Part model, mm, in its own coordinate system. Face numbers are marked on the shaded views. A direction names the side the tool comes from. Give positions to 0.01 mm unless a question says otherwise; leave off trailing zeros. Write each loop counter-clockwise with the first axis right and the second up, starting at its lowest first coordinate (ties: lowest second). Pieces come first, ordered by that corner, then holes. Notation, with made-up numbers: (9, 78) - (26, 78) arc R20 cw to (26, 115) - close; hole circle Ø11 at (-25, 27). An arc over 180 degrees is marked (long way). Answer as a JSON object with one key per item and string values. Group by question number.
```python
from build123d import *

# Parameters (mm, degrees)
SKETCH1_W                     = 196.85
SKETCH1_H                     = 152.4
SKETCH1_W_2                   = 146.05
SKETCH1_H_2                   = 101.6
BOSS_EXTRUDE1_DEPTH           = 1.5875
EDGE_FLANGE1_STRIP_W          = 26.35
EDGE_FLANGE1_STRIP_H          = 1.5875
EDGE_FLANGE1_STRIP_CUT_DEPTH  = 152.4
EDGE_FLANGE1_DEPTH            = 152.4
EDGE_FLANGE2_STRIP_W          = 26.35
EDGE_FLANGE2_STRIP_H          = 1.5875
EDGE_FLANGE2_STRIP_CUT_DEPTH  = 152.4
EDGE_FLANGE2_DEPTH            = 152.4
SKETCH16_W                    = 146.05
SKETCH16_H                    = 101.6
CUT_EXTRUDE1_DEPTH            = 1.5875
SKETCH17_W                    = 31.75
SKETCH17_H                    = 114.3
CUT_EXTRUDE2_DEPTH            = 1.5875
SKETCH25_W                    = 1.5875
SKETCH25_H                    = 101.6
CUT_EXTRUDE3_DEPTH            = 0.0254
EDGE_FLANGE5_STRIP_W          = 26.35
EDGE_FLANGE5_STRIP_H          = 1.5875
EDGE_FLANGE5_STRIP_CUT_DEPTH  = 25.4
EDGE_FLANGE5_RELIEF_W         = 27.14375
EDGE_FLANGE5_RELIEF_H         = 0.79375
EDGE_FLANGE5_RELIEF_CUT_DEPTH = 1.5875
EDGE_FLANGE5_DEPTH            = 25.4
EDGE_FLANGE6_STRIP_W          = 26.35
EDGE_FLANGE6_STRIP_H          = 1.5875
EDGE_FLANGE6_STRIP_CUT_DEPTH  = 25.4
EDGE_FLANGE6_RELIEF_W         = 27.14375
EDGE_FLANGE6_RELIEF_H         = 0.79375
EDGE_FLANGE6_RELIEF_CUT_DEPTH = 1.5875
EDGE_FLANGE6_DEPTH            = 25.4
SKETCH32_R                    = 3.175
CUT_EXTRUDE4_DEPTH            = 10.16
SKETCH33_R                    = 3.175
CUT_EXTRUDE5_DEPTH            = 10.16
FILLET1_R                     = 2.54
FILLET2_R                     = 2.54
FILLET3_R                     = 2.54
SKETCH35_W                    = 1.5875
SKETCH35_H                    = 101.6
CUT_EXTRUDE6_DEPTH            = 0.0254
EDGE_FLANGE7_STRIP_W          = 26.35
EDGE_FLANGE7_STRIP_H          = 1.5875
EDGE_FLANGE7_STRIP_CUT_DEPTH  = 25.4
EDGE_FLANGE7_RELIEF_W         = 27.14375
EDGE_FLANGE7_RELIEF_H         = 0.79375
EDGE_FLANGE7_RELIEF_CUT_DEPTH = 1.5875
EDGE_FLANGE7_DEPTH            = 25.4
EDGE_FLANGE8_STRIP_W          = 26.35
EDGE_FLANGE8_STRIP_H          = 1.5875
EDGE_FLANGE8_STRIP_CUT_DEPTH  = 25.4
EDGE_FLANGE8_RELIEF_W         = 27.14375
EDGE_FLANGE8_RELIEF_H         = 0.79375
EDGE_FLANGE8_RELIEF_CUT_DEPTH = 1.5875
EDGE_FLANGE8_DEPTH            = 25.4
SKETCH42_R                    = 3.175
CUT_EXTRUDE7_DEPTH            = 10.16
SKETCH43_R                    = 3.175
CUT_EXTRUDE8_DEPTH            = 10.16


# Sheet-metal steps are written as plain solids
with BuildPart() as part:
    # Sketch1 → Boss-Extrude1 (new body)
    with BuildSketch(Plane.XY):
        with Locations((-98.425, 76.2)):
            Rectangle(SKETCH1_W, SKETCH1_H)
        with Locations((-98.425, 76.2)):
            Rectangle(SKETCH1_W_2, SKETCH1_H_2, mode=Mode.SUBTRACT)
    extrude(amount=BOSS_EXTRUDE1_DEPTH)

    # Edge-Flange1 strip (across the edge) → Edge-Flange1 strip cut (cut)
    with BuildSketch(Plane(origin=(0, 152.4, 0), x_dir=(-1, 0, 0), z_dir=(0, -1, 0))):
        with Locations((-1.5875, -0.79375)):
            Rectangle(EDGE_FLANGE1_STRIP_W, EDGE_FLANGE1_STRIP_H)
    extrude(amount=EDGE_FLANGE1_STRIP_CUT_DEPTH, mode=Mode.SUBTRACT)

    # Edge-Flange1 section (across the edge) → Edge-Flange1 (add)
    with BuildSketch(Plane(origin=(0, 152.4, 0), x_dir=(-1, 0, 0), z_dir=(0, -1, 0))):
        with BuildLine():
            Line((0, 10), (0, 80.9625))
            Line((0, 80.9625), (1.5875, 80.9625))
            Line((1.5875, 80.9625), (1.5875, 10))
            ThreePointArc((1.5875, 10), (4.516432188, 2.928932188), (11.5875, 0))
            Line((11.5875, 0), (11.5875, -1.5875))
            ThreePointArc((11.5875, -1.5875), (3.393900173, 1.806400173), (0, 10))
        make_face()
    extrude(amount=EDGE_FLANGE1_DEPTH)

    # Edge-Flange2 strip (across the edge) → Edge-Flange2 strip cut (cut)
    with BuildSketch(Plane(origin=(-1.5875, 152.4, -80.9625), x_dir=(0, 0, 1), z_dir=(0, -1, 0))):
        with Locations((-1.5875, -0.79375)):
            Rectangle(EDGE_FLANGE2_STRIP_W, EDGE_FLANGE2_STRIP_H)
    extrude(amount=EDGE_FLANGE2_STRIP_CUT_DEPTH, mode=Mode.SUBTRACT)

    # Edge-Flange2 section (across the edge) → Edge-Flange2 (add)
    with BuildSketch(Plane(origin=(-1.5875, 152.4, -80.9625), x_dir=(0, 0, 1), z_dir=(0, -1, 0))):
        with BuildLine():
            Line((0, 10), (0, 195.2625))
            Line((0, 195.2625), (1.5875, 195.2625))
            Line((1.5875, 195.2625), (1.5875, 10))
            ThreePointArc((1.5875, 10), (4.516432188, 2.928932188), (11.5875, 0))
            Line((11.5875, 0), (11.5875, -1.5875))
            ThreePointArc((11.5875, -1.5875), (3.393900173, 1.806400173), (0, 10))
        make_face()
    extrude(amount=EDGE_FLANGE2_DEPTH)

    # Sketch16 → Cut-Extrude1 (cut)
    with BuildSketch(Plane(origin=(0, 0, -80.9625), x_dir=(-1, 0, 0), z_dir=(0, 0, -1))):
        with Locations((98.425, 76.2)):
            Rectangle(SKETCH16_W, SKETCH16_H)
    extrude(amount=-CUT_EXTRUDE1_DEPTH, mode=Mode.SUBTRACT)

    # Sketch17 → Cut-Extrude2 (cut)
    with BuildSketch(Plane.ZY.offset(1.5875)):
        with Locations((-39.6875, 76.2)):
            Rectangle(SKETCH17_W, SKETCH17_H)
    extrude(amount=-CUT_EXTRUDE2_DEPTH, mode=Mode.SUBTRACT)

    # Sketch25 → Cut-Extrude3 (cut)
    with BuildSketch(Plane.ZY.offset(196.85)):
        with Locations((-80.16875, 76.2)):
            Rectangle(SKETCH25_W, SKETCH25_H)
    extrude(amount=-CUT_EXTRUDE3_DEPTH, mode=Mode.SUBTRACT)

    # Edge-Flange5 strip (across the edge) → Edge-Flange5 strip cut (cut)
    with BuildSketch(Plane(origin=(-196.85, 152.4, -79.375), x_dir=(1, 0, 0), z_dir=(0, -1, 0))):
        with Locations((-1.5875, -0.79375)):
            Rectangle(EDGE_FLANGE5_STRIP_W, EDGE_FLANGE5_STRIP_H)
    extrude(amount=EDGE_FLANGE5_STRIP_CUT_DEPTH, mode=Mode.SUBTRACT)

    # Edge-Flange5 relief (on the sheet) → Edge-Flange5 relief cut (cut)
    with BuildSketch(Plane(origin=(-185.2625, 152.4, -79.375), x_dir=(1, 0, 0), z_dir=(0, 0, 1))):
        with Locations((-12.778125, -25.796875)):
            Rectangle(EDGE_FLANGE5_RELIEF_W, EDGE_FLANGE5_RELIEF_H)
    extrude(amount=-EDGE_FLANGE5_RELIEF_CUT_DEPTH, mode=Mode.SUBTRACT)

    # Edge-Flange5 section (across the edge) → Edge-Flange5 (add)
    with BuildSketch(Plane(origin=(-196.85, 152.4, -79.375), x_dir=(1, 0, 0), z_dir=(0, -1, 0))):
        with BuildLine():
            Line((0, 10), (0, 23.8125))
            Line((0, 23.8125), (1.5875, 23.8125))
            Line((1.5875, 23.8125), (1.5875, 10))
            ThreePointArc((1.5875, 10), (4.516432188, 2.928932188), (11.5875, 0))
            Line((11.5875, 0), (11.5875, -1.5875))
            ThreePointArc((11.5875, -1.5875), (3.393900173, 1.806400173), (0, 10))
        make_face()
    extrude(amount=EDGE_FLANGE5_DEPTH)

    # Edge-Flange6 strip (across the edge) → Edge-Flange6 strip cut (cut)
    with BuildSketch(Plane(origin=(-196.85, 25.4, -79.375), x_dir=(1, 0, 0), z_dir=(0, -1, 0))):
        with Locations((-1.5875, -0.79375)):
            Rectangle(EDGE_FLANGE6_STRIP_W, EDGE_FLANGE6_STRIP_H)
    extrude(amount=EDGE_FLANGE6_STRIP_CUT_DEPTH, mode=Mode.SUBTRACT)

    # Edge-Flange6 relief (on the sheet) → Edge-Flange6 relief cut (cut)
    with BuildSketch(Plane(origin=(-185.2625, 25.4, -79.375), x_dir=(1, 0, 0), z_dir=(0, 0, 1))):
        with Locations((-12.778125, 0.396875)):
            Rectangle(EDGE_FLANGE6_RELIEF_W, EDGE_FLANGE6_RELIEF_H)
    extrude(amount=-EDGE_FLANGE6_RELIEF_CUT_DEPTH, mode=Mode.SUBTRACT)

    # Edge-Flange6 section (across the edge) → Edge-Flange6 (add)
    with BuildSketch(Plane(origin=(-196.85, 25.4, -79.375), x_dir=(1, 0, 0), z_dir=(0, -1, 0))):
        with BuildLine():
            Line((0, 10), (0, 23.8125))
            Line((0, 23.8125), (1.5875, 23.8125))
            Line((1.5875, 23.8125), (1.5875, 10))
            ThreePointArc((1.5875, 10), (4.516432188, 2.928932188), (11.5875, 0))
            Line((11.5875, 0), (11.5875, -1.5875))
            ThreePointArc((11.5875, -1.5875), (3.393900173, 1.806400173), (0, 10))
        make_face()
    extrude(amount=EDGE_FLANGE6_DEPTH)

    # Sketch32 → Cut-Extrude4 (cut)
    with BuildSketch(Plane.ZY.offset(196.85)):
        with Locations((-61.9125, 146.05)):
            Circle(SKETCH32_R)
        with Locations((-61.9125, 133.35)):
            Circle(SKETCH32_R)
    extrude(amount=-CUT_EXTRUDE4_DEPTH, mode=Mode.SUBTRACT)

    # Sketch33 → Cut-Extrude5 (cut)
    with BuildSketch(Plane.ZY.offset(196.85)):
        with Locations((-61.9125, 19.05)):
            Circle(SKETCH33_R)
        with Locations((-61.9125, 6.35)):
            Circle(SKETCH33_R)
    extrude(amount=-CUT_EXTRUDE5_DEPTH, mode=Mode.SUBTRACT)

    # Fillet1
    fillet1_edges = [part.edges().sort_by_distance(p)[0] for p in [
        (-25.4, 127, 0.79375),
    ]]
    fillet(fillet1_edges, radius=FILLET1_R)

    # Fillet2
    fillet2_edges = [part.edges().sort_by_distance(p)[0] for p in [
        (-171.45, 25.4, 0.79375),
        (-25.4, 25.4, 0.79375),
        (-171.45, 127, 0.79375),
        (-25.4, 25.4, -80.16875),
        (-25.4, 127, -80.16875),
        (-171.45, 127, -80.16875),
    ]]
    fillet(fillet2_edges, radius=FILLET2_R)

    # Fillet3
    fillet3_edges = [part.edges().sort_by_distance(p)[0] for p in [
        (-0.79375, 19.05, -55.5625),
        (-0.79375, 133.35, -55.5625),
        (-0.79375, 133.35, -23.8125),
        (-0.79375, 19.05, -23.8125),
        (-171.45, 25.4, -80.16875),
    ]]
    fillet(fillet3_edges, radius=FILLET3_R)

    # Sketch35 → Cut-Extrude6 (cut)
    with BuildSketch(Plane.ZY.offset(196.85)):
        with Locations((0.79375, 76.2)):
            Rectangle(SKETCH35_W, SKETCH35_H)
    extrude(amount=-CUT_EXTRUDE6_DEPTH, mode=Mode.SUBTRACT)

    # Edge-Flange7 strip (across the edge) → Edge-Flange7 strip cut (cut)
    with BuildSketch(Plane(origin=(-196.85, 152.4, 1.5875), x_dir=(1, 0, 0), z_dir=(0, -1, 0))):
        with Locations((-1.5875, -0.79375)):
            Rectangle(EDGE_FLANGE7_STRIP_W, EDGE_FLANGE7_STRIP_H)
    extrude(amount=EDGE_FLANGE7_STRIP_CUT_DEPTH, mode=Mode.SUBTRACT)

    # Edge-Flange7 relief (on the sheet) → Edge-Flange7 relief cut (cut)
    with BuildSketch(Plane(origin=(-185.2625, 152.4, 1.5875), x_dir=(1, 0, 0), z_dir=(0, 0, 1))):
        with Locations((-12.778125, -25.796875)):
            Rectangle(EDGE_FLANGE7_RELIEF_W, EDGE_FLANGE7_RELIEF_H)
    extrude(amount=-EDGE_FLANGE7_RELIEF_CUT_DEPTH, mode=Mode.SUBTRACT)

    # Edge-Flange7 section (across the edge) → Edge-Flange7 (add)
    with BuildSketch(Plane(origin=(-196.85, 152.4, 1.5875), x_dir=(1, 0, 0), z_dir=(0, -1, 0))):
        with BuildLine():
            Line((0, 10), (0, 23.8125))
            Line((0, 23.8125), (1.5875, 23.8125))
            Line((1.5875, 23.8125), (1.5875, 10))
            ThreePointArc((1.5875, 10), (4.516432188, 2.928932188), (11.5875, 0))
            Line((11.5875, 0), (11.5875, -1.5875))
            ThreePointArc((11.5875, -1.5875), (3.393900173, 1.806400173), (0, 10))
        make_face()
    extrude(amount=EDGE_FLANGE7_DEPTH)

    # Edge-Flange8 strip (across the edge) → Edge-Flange8 strip cut (cut)
    with BuildSketch(Plane(origin=(-196.85, 25.4, 1.5875), x_dir=(1, 0, 0), z_dir=(0, -1, 0))):
        with Locations((-1.5875, -0.79375)):
            Rectangle(EDGE_FLANGE8_STRIP_W, EDGE_FLANGE8_STRIP_H)
    extrude(amount=EDGE_FLANGE8_STRIP_CUT_DEPTH, mode=Mode.SUBTRACT)

    # Edge-Flange8 relief (on the sheet) → Edge-Flange8 relief cut (cut)
    with BuildSketch(Plane(origin=(-185.2625, 25.4, 1.5875), x_dir=(1, 0, 0), z_dir=(0, 0, 1))):
        with Locations((-12.778125, 0.396875)):
            Rectangle(EDGE_FLANGE8_RELIEF_W, EDGE_FLANGE8_RELIEF_H)
    extrude(amount=-EDGE_FLANGE8_RELIEF_CUT_DEPTH, mode=Mode.SUBTRACT)

    # Edge-Flange8 section (across the edge) → Edge-Flange8 (add)
    with BuildSketch(Plane(origin=(-196.85, 25.4, 1.5875), x_dir=(1, 0, 0), z_dir=(0, -1, 0))):
        with BuildLine():
            Line((0, 10), (0, 23.8125))
            Line((0, 23.8125), (1.5875, 23.8125))
            Line((1.5875, 23.8125), (1.5875, 10))
            ThreePointArc((1.5875, 10), (4.516432188, 2.928932188), (11.5875, 0))
            Line((11.5875, 0), (11.5875, -1.5875))
            ThreePointArc((11.5875, -1.5875), (3.393900173, 1.806400173), (0, 10))
        make_face()
    extrude(amount=EDGE_FLANGE8_DEPTH)

    # Sketch42 → Cut-Extrude7 (cut)
    with BuildSketch(Plane.ZY.offset(196.85)):
        with Locations((19.05, 146.05)):
            Circle(SKETCH42_R)
        with Locations((19.05, 133.35)):
            Circle(SKETCH42_R)
    extrude(amount=-CUT_EXTRUDE7_DEPTH, mode=Mode.SUBTRACT)

    # Sketch43 → Cut-Extrude8 (cut)
    with BuildSketch(Plane.ZY.offset(196.85)):
        with Locations((19.05, 19.05)):
            Circle(SKETCH43_R)
        with Locations((19.05, 6.35)):
            Circle(SKETCH43_R)
    extrude(amount=-CUT_EXTRUDE8_DEPTH, mode=Mode.SUBTRACT)


solid = part.part
```
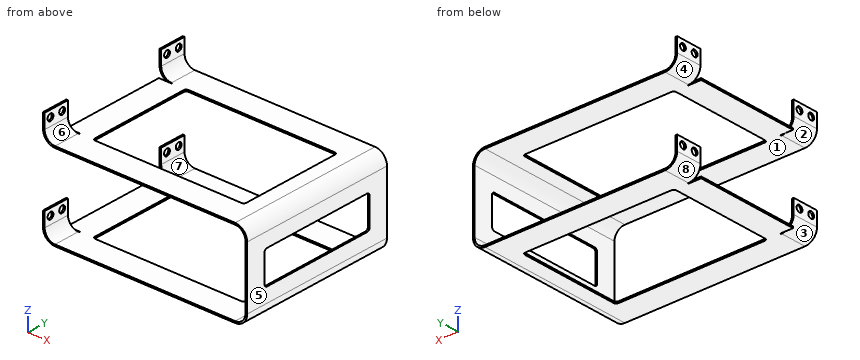
1) Band-saw the part on D-D (z = -39). List the corners of the cut face in (x, y).
2) Band-saw the part on B-B (z = 19.05). State how many separate pieces and enclosed holes the cut face has, plus the area to 3 significant figures.
3) Probe line 1 (Z direction, x = -11, y = 72); line 2 (X direction, y = 145, z = -69); line 3 (Z direction, x = -195.65, y = 133.35) (1 decimal). List the from-to ranges inside material, lowest first.
4) Which spindle directions (+Z, -Z, +X, -X, +Y, -Y) get a long thin tool onto all of the face, cutting with end or side? Do the marked faces 1, 2, 3 and 4. Say none if no direction does.
5) Band-saw the part on A-A (x = -136.5). List the corners of the cut face in (y, z) (1 decimal).
6) Mould opens along Z. For the marked faces 5, 6, 7 and 8 say: pulls with the +Z half, pulls with the -Z half, needs draft (parallel to the pull), parting line crosses it, or undercut.
7) Drop flat-ended pins along their axis: P1, Ø4, axis at y = 131.5, z = -20.5, coming from the -X side; P2, Ø15, axis at y = 16, z = 19, coming from the +X side; P3, Ø1.3, axis at x = -0.5, y = 71, coming from the +Z side. Give the stop position or say it passes through.
Verdict:
{
 "1": {"outline": "(-1.59, 0) - (0, 0) - (0, 19.05) - (-1.59, 19.05) - close; (-1.59, 133.35) - (0, 133.35) - (0, 152.4) - (-1.59, 152.4) - close"},
 "2": {"separate pieces": "6", "enclosed holes": "0", "area": "40.3 mm2"},
 "3": {"line 1": "-80.95 to -79.36, -0.02 to 1.57", "line 2": "-196.85 to -195.26, -1.59 to 0", "line 3": "-74.5 to -65.1, -58.7 to -55.6, 6.5 to 15.9, 22.2 to 25.4"},
 "4": {"face 1": "-X, +Y, -Y", "face 2": "-X, -Y", "face 3": "-Z, -X, -Y", "face 4": "-X, +Y"},
 "5": {"outline": "(0, -81) - (25.4, -81) - (25.4, -79.4) - (0, -79.4) - close; (0, 0) - (25.4, 0) - (25.4, 1.6) - (0, 1.6) - close; (127, -81) - (152.4, -81) - (152.4, -79.4) - (127, -79.4) - close; (127, 0) - (152.4, 0) - (152.4, 1.6) - (127, 1.6) - close"},
 "6": {"face 5": "needs draft", "face 6": "pulls with the +Z half", "face 7": "undercut", "face 8": "pulls with the -Z half"},
 "7": {"P1": "x = -1.59", "P2": "x = -195.26", "P3": "z = -4.97"}
}
